Read the model definition and answer for the solid it produces. Units are mm, in the model's axes. A direction names the side the tool comes from. Coordinates: 2 decimals unless noted, no trailing zeros. Write each loop counter-clockwise with the first axis right and the second up, starting at its lowest first coordinate (ties: lowest second). Pieces come first, ordered by that corner, then holes. Notation, with made-up numbers: (34.5, 62) -> (78.5, 62) arc R12 cw to (78.5, 76) -> close; hole circle Ø10 at (34.5, -17.5). An arc over 180 degrees is marked (long way). Answer in a Markdown table with one row per item. Add a question column.
Item 1: Which of the six approach directions +Z, -Z, +X, -X, +Y, -Y give full straight-line access (tool end or side, diameter ignored) to faces 4 (the face through (-5.506, 18.806, -24.796)), 5 (the face through (21, -1.588, 1))?
Item 2: Section B-B on z = 0 is taken. Write down the section's boundary in (x, y).
Item 3: Section C-C on y = 12 is taken. Write down the section's boundary in (x, z), then the cut area to 3 significant figures.
Item 4: For a pull along Z with two mould halves and no side action, classify faces 1 (the face through (21, 1.588, -21)), 2 (the face through (-22.025, -0.022, -99.184)), 3 (the face through (2.75, 17.73, -12.4)) as +Z half, -Z half, draft (parallel to the pull), parting line (faces both ways), or undercut.
Item 5: Section A-A on x = 0 is taken. Write down the section's boundary in (y, z).
Item 6: Section D-D on z = -21 is taken. Write down the section's boundary in (x, y), then the cut area to 3 significant figures.
Item 7: Given pin 1 Ø10 at (x, y) = (-13.5, 7) entering from -Z; pin 2 Ø6 at (y, z) = (4, -23.5) entering from +X, each flat-ended and moving along its own axis, determine where each tip first touches the part or whether it passes through.
Item 8: Straight lines are drawn through the part: line 1 (Z direction, x = 0, y = 6); line 2 (Y direction, x = -39, z = -2); line 3 (X direction, y = 3, z = -11.5). For each, find the intervals that lie inside material, in ascending order. Write a range as from..to.
```python
from build123d import *

# Parameters (mm, degrees)
F0_R     = 101.6
F1_DEPTH = 1.5875
F2_R     = 25.4
F3_DEPTH = 38.1
F4_R     = 12.7
F5_DEPTH = 63.5
F6_R     = 12.7
F7_DEPTH = 63.5


with BuildPart() as f1:
    # F0 (on Front) → F1 (new body, symmetric)
    with BuildSketch(Plane.XZ):
        Circle(F0_R)
    extrude(amount=F1_DEPTH, both=True)

    # F2 (on face) → F3 (join)
    with BuildSketch(Plane.XZ.offset(1.5875)):
        Circle(F2_R)
    extrude(amount=-F3_DEPTH)

    # F4 (on face) → F5 (cut)
    with BuildSketch(Plane(origin=(0, 36.5125, 0), x_dir=(-1, 0, 0), z_dir=(0, 1, 0))):
        Circle(F4_R)
    extrude(amount=F5_DEPTH, mode=Mode.SUBTRACT)

    # F6 (on face) → F7 (cut)
    with BuildSketch(Plane(origin=(0, 36.5125, 0), x_dir=(-1, 0, 0), z_dir=(0, 1, 0))):
        Circle(F6_R)
    extrude(amount=-F7_DEPTH, mode=Mode.SUBTRACT)


solid = f1.part
```
Results below:
| question | item | result |
|---|---|---|
| 1 | face 4 | +Y |
| 1 | face 5 | +Z, -Z, +X, -X, -Y |
| 2 | outline | (-101.6, -1.59) -> (-12.7, -1.59) -> (-12.7, 36.51) -> (-25.4, 36.51) -> (-25.4, 1.59) -> (-101.6, 1.59) -> close; (12.7, -1.59) -> (101.6, -1.59) -> (101.6, 1.59) -> (25.4, 1.59) -> (25.4, 36.51) -> (12.7, 36.51) -> close |
| 3 | outline | circle Ø50.8 at (0, 0); hole circle Ø25.4 at (0, 0) |
| 3 | area | 1,520 mm2 |
| 4 | face 1 | draft |
| 4 | face 2 | parting line |
| 4 | face 3 | undercut |
| 5 | outline | (-1.59, -101.6) -> (1.59, -101.6) -> (1.59, -25.4) -> (36.51, -25.4) -> (36.51, -12.7) -> (-1.59, -12.7) -> close; (-1.59, 12.7) -> (36.51, 12.7) -> (36.51, 25.4) -> (1.59, 25.4) -> (1.59, 101.6) -> (-1.59, 101.6) -> close |
| 6 | outline | (-99.41, -1.59) -> (99.41, -1.59) -> (99.41, 1.59) -> (14.29, 1.59) -> (14.29, 36.51) -> (-14.29, 36.51) -> (-14.29, 1.59) -> (-99.41, 1.59) -> close |
| 6 | area | 1,630 mm2 |
| 7 | pin 1 | stops at z = -23.94 |
| 7 | pin 2 | stops at x = 99.25 |
| 8 | line 1 | z = -25.4..-12.7, 12.7..25.4 |
| 8 | line 2 | y = -1.59..1.59 |
| 8 | line 3 | x = -22.65..-5.39, 5.39..22.65 |
